Here's how the part is built. I have some questions about the finished solid (model axes, mm). A direction names the side the tool comes from. Round coordinates to 2 decimals unless told otherwise and drop trailing zeros. Write each loop counter-clockwise with the first axis right and the second up, starting at its lowest first coordinate (ties: lowest second). Pieces come first, ordered by that corner, then holes. Notation, with made-up numbers: (22.5, 68) -> (61.5, 68) arc R29 cw to (61.5, 96) -> close; hole circle Ø1 at (-4.5, -13). An arc over 180 degrees is marked (long way). Answer as CSV lines item,"result".
```python
from build123d import *

# Parameters (mm, degrees)
SKETCH_1_R          = 1.6
EXTRUDE_1_DEPTH     = 1.2
EXTRUDE_2_DEPTH     = 8
SKETCH_3_R          = 1.6
CUT_EXTRUDE_1_DEPTH = 8


with BuildPart() as part:
    # 草图1 → 凸台-拉伸1 (new body)
    with BuildSketch(Plane(origin=(0, 0, 0), x_dir=(1, 0, 0), z_dir=(0, 1, 0))):
        with BuildLine():
            Line((15.45, 0), (15.45, 21.5))
            ThreePointArc((15.45, 21.5), (26.5, 32.55), (37.55, 21.5))
            Line((37.55, 21.5), (37.55, 0))
            Line((37.55, 0), (53, 0))
            Line((53, 0), (53, 66.5))
            Line((53, 66.5), (0, 66.5))
            Line((0, 66.5), (0, 0))
            Line((0, 0), (15.45, 0))
        make_face()
        with Locations(Location((11, 6, 0), (0, 0, 270))):
            Circle(SKETCH_1_R, mode=Mode.SUBTRACT)
        with Locations(Location((11, 37, 0), (0, 0, 270))):
            Circle(SKETCH_1_R, mode=Mode.SUBTRACT)
        with Locations(Location((42, 37, 0), (0, 0, 90))):
            Circle(SKETCH_1_R, mode=Mode.SUBTRACT)
        with Locations(Location((42, 6, 0), (0, 0, 90))):
            Circle(SKETCH_1_R, mode=Mode.SUBTRACT)
    extrude(amount=EXTRUDE_1_DEPTH)

    # 草图2 → 凸台-拉伸2 (add)
    with BuildSketch(Plane.XZ):
        Polygon((1, 0), (1, -65.5), (52, -65.5), (52, 0), (53, 0), (53, -66.5), (0, -66.5), (0, 0), align=None)
    extrude(amount=EXTRUDE_2_DEPTH)

    # 草图3 → 切除-拉伸1 (cut)
    with BuildSketch(Plane(origin=(0, 0, -66.5), x_dir=(-1, 0, 0), z_dir=(0, 0, -1))):
        with Locations((-11.5, -4)):
            Circle(SKETCH_3_R)
        with Locations((-41.5, -4)):
            Circle(SKETCH_3_R)
    extrude(amount=-CUT_EXTRUDE_1_DEPTH, mode=Mode.SUBTRACT)


solid = part.part
```
1. Suppose I cut it at D-D on z = -26. Please give me the cut outline in (x, y).
Numbers:
outline,"(0, -8) -> (1, -8) -> (1, 0) -> (16.41, 0) -> (16.41, 1.2) -> (0, 1.2) -> close; (36.59, 0) -> (52, 0) -> (52, -8) -> (53, -8) -> (53, 1.2) -> (36.59, 1.2) -> close"
2. Suppose I cut it at C-C on x = 11. Please give me the cut outline in (y, z), and give its area (3 significant figures).
Numbers:
outline,"(-8, -66.5) -> (-5.52, -66.5) -> (-5.52, -65.5) -> (-8, -65.5) -> close; (-2.48, -66.5) -> (1.2, -66.5) -> (1.2, -38.6) -> (0, -38.6) -> (0, -65.5) -> (-2.48, -65.5) -> close; (0, -35.4) -> (1.2, -35.4) -> (1.2, -7.6) -> (0, -7.6) -> close; (0, -4.4) -> (1.2, -4.4) -> (1.2, 0) -> (0, 0) -> close"
area,"77.1 mm^2"
3. For pin 1 Ø15.5 at (x, z) = (16.5, -29) entering from -Y; pin 2 Ø3 at (x, z) = (42, -6) entering from +Y; pin 3 Ø4 at (x, y) = (29, -2.5) entering from +Z, each with a flat end and sliding along its axis, tell me the tip position at first contact or that it passes through.
Numbers:
pin 1,"stops at y = 0"
pin 2,"passes through"
pin 3,"stops at z = -65.5"
4. If I drill on line 1 (Z direction, x = 42, y = 0.45); line 2 (X direction, y = 0.55, z = -37); line 3 (X direction, y = -1.75, z = -16.5), over which ranges is the centre line in solid material (lowest first)?
Numbers:
line 1,"z = -66.5 to -38.6, -35.4 to -7.6, -4.4 to 0"
line 2,"x = 0 to 9.4, 12.6 to 40.4, 43.6 to 53"
line 3,"x = 0 to 1, 52 to 53"
5. Suppose I cut it at A-A on y = -4. Please give me the cut outline in (x, z), and give its area (3 significant figures).
Numbers:
outline,"(0, -66.5) -> (9.9, -66.5) -> (9.9, -65.5) -> (1, -65.5) -> (1, 0) -> (0, 0) -> close; (13.1, -66.5) -> (39.9, -66.5) -> (39.9, -65.5) -> (13.1, -65.5) -> close; (43.1, -66.5) -> (53, -66.5) -> (53, 0) -> (52, 0) -> (52, -65.5) -> (43.1, -65.5) -> close"
area,"178 mm^2"
6. On a 3-axis mill with a long thin cutter (end or side, diameter ignored), from which of +Z, -Z, +X, -X, +Y, -Y can I reach the whole of each face in a straight line? I mean faces 1 (the face through (11.481, 0.592, -4.474)), 2 (the face through (1, -4, -32)). Say none if no direction works.
Numbers:
face 1,"+Y, -Y"
face 2,"+Z, -Y"
7. Suppose I cut it at B-B on z = -6. Please give me the cut outline in (x, y).
Numbers:
outline,"(0, -8) -> (1, -8) -> (1, 0) -> (9.4, 0) -> (9.4, 1.2) -> (0, 1.2) -> close; (12.6, 0) -> (15.45, 0) -> (15.45, 1.2) -> (12.6, 1.2) -> close; (37.55, 0) -> (40.4, 0) -> (40.4, 1.2) -> (37.55, 1.2) -> close; (43.6, 0) -> (52, 0) -> (52, -8) -> (53, -8) -> (53, 1.2) -> (43.6, 1.2) -> close"
8. If we mould it in two halves opening along Z, with no side actions, what happens to faces 3 (the face through (12.08, 0.59, -38.18)), 4 (the face through (26, -4, -65.5)), 5 (the face through (26, 0, -40))? For each: released by +Z, released by -Z, zero draft, split by the parting line, or undercut.
Numbers:
face 3,"undercut"
face 4,"released by +Z"
face 5,"zero draft"
